from build123d import *

# Parameters (mm, degrees)
F0_R     = 5
F1_DEPTH = 10
F2_R     = 1.25
F3_DEPTH = 3.5
F4_R     = 10
F4_R_2   = 1.5
F4_R_3   = 5
F5_DEPTH = 3


with BuildPart() as f1:
    # F0 (on Top) → F1 (new body)
    with BuildSketch(Plane.XY):
        Circle(F0_R)
        with BuildLine():
            ThreePointArc((1.5, 2), (2.2360679775, 1.1180339887), (2.5, 0))
            ThreePointArc((2.5, 0), (2.2360679775, -1.1180339887), (1.5, -2))
            ThreePointArc((1.5, -2), (-2.5, 0), (1.5, 2))
        make_face(mode=Mode.SUBTRACT)
        with BuildLine():
            ThreePointArc((1.5, -2), (2.2360679775, -1.1180339887), (2.5, 0))
            ThreePointArc((2.5, 0), (2.2360679775, 1.1180339887), (1.5, 2))
            Line((1.5, 2), (1.5, -2))
        make_face()
    extrude(amount=F1_DEPTH)

    # F2 (on face) → F3 (cut, through all)
    with BuildSketch(Plane(origin=(1.5, 0, 0), x_dir=(0, -1, 0), z_dir=(-1, 0, 0))):
        with Locations((0, 5)):
            Circle(F2_R)
    extrude(amount=-F3_DEPTH, mode=Mode.SUBTRACT)

    # F4 (on face) → F5 (join)
    with BuildSketch(Plane.XY.offset(10)):
        Circle(F4_R)
        with Locations((0, -7.5)):
            Circle(F4_R_2, mode=Mode.SUBTRACT)
        with Locations((-7.5, 0)):
            Circle(F4_R_2, mode=Mode.SUBTRACT)
        Circle(F4_R_3, mode=Mode.SUBTRACT)
        with Locations((7.5, 0)):
            Circle(F4_R_2, mode=Mode.SUBTRACT)
        with Locations((0, 7.5)):
            Circle(F4_R_2, mode=Mode.SUBTRACT)
        Circle(F4_R_3)
        with BuildLine():
            Line((1.5, 2), (1.5, -2))
            ThreePointArc((1.5, -2), (-2.5, 0), (1.5, 2))
        make_face(mode=Mode.SUBTRACT)
        with BuildLine():
            ThreePointArc((1.5, 2), (-2.5, 0), (1.5, -2))
            Line((1.5, -2), (1.5, 2))
        make_face()
    extrude(amount=F5_DEPTH)


solid = f1.part
Verification items for the finished model (mm, model axes). A direction names the side the tool comes from. Give positions to 0.01 mm unless a question says otherwise; leave off trailing zeros. Order: outer loops, then holes, each group sorted by start corner. A loop starts at its lowest first (then second) coordinate and runs counter-clockwise, first axis right, second up. Notation, with made-up numbers: M 7.25,75.5 L 18.25,75.5 A17 cw 18.25,93.5 Z; hole C 87,72 d1. An arc over 180 degrees is marked long. Answer as a JSON object with one key per item and string values. Group by question number.
1) Mould release check, pull along X, two halves, no side actions. Record for faces 4 (the face through (-1.08, -4.88, 4.93)), 5 (the face through (-1, 0, 10)), 6 (the face through (2, 5, 10)): released by +X, released by -X, zero draft, split by the parting line, or undercut.
2) Cross-section at D-D (x = 8.5). Enter the section's corners in (y, z).
3) Cross-section at C-C (y = -8). Enter the section's corners in (x, z).
4) Access from +Z, -Z, +X, -X, +Y, -Y to the whole of each face (thin tool, end or side, straight path). Record for faces 1 (the face through (6, 0, 11)), 2 (the face through (3.23, 0.27, 3.78)), 3 (the face through (1.5, 1.4, 4.9)).
5) Depth check by flat-ended pin: pin 1 Ø2.5 at (x, y) = (0, 7.5) entering from +Z; pin 2 Ø3 at (x, y) = (-0.5, 0.5) entering from -Z; pin 3 Ø2 at (y, z) = (-2, 11) entering from -X; pin 4 Ø1.5 at (x, z) = (4.5, 2.5) entering from +Y. Enter the tip coordinate at first touch or a pass-through.
6) Scan lines: line 1 along Y through (x, z) = (0, 12.3); line 2 along X through (y, z) = (-0.75, 10.5); line 3 along X through (y, z) = (-0.5, 10.5). Record each from-to range of solid material in increasing order. Write a range as [from, to].
7) Cross-section at A-A (x = 0). Enter the section's corners in (y, z), then the cut area to 3 significant figures.
8) Cross-section at B-B (y = 0). Enter the section's corners in (x, z).
Result sheet:
{
 "1": {"face 4": "split by the parting line", "face 5": "undercut", "face 6": "zero draft"},
 "2": {"outline": "M -5.27,10 L -1.12,10 L -1.12,13 L -5.27,13 Z; M 1.12,10 L 5.27,10 L 5.27,13 L 1.12,13 Z"},
 "3": {"outline": "M -6,10 L -1.41,10 L -1.41,13 L -6,13 Z; M 1.41,10 L 6,10 L 6,13 L 1.41,13 Z"},
 "4": {"face 1": "+Z, -Z", "face 2": "+X", "face 3": "-Z"},
 "5": {"pin 1": "passes through", "pin 2": "stops at z = 10", "pin 3": "stops at x = -9.95", "pin 4": "stops at y = 3.31"},
 "6": {"line 1": "y = [-10, -9], [-6, 6], [9, 10]", "line 2": "x = [-9.97, -8.8], [-6.2, 6.2], [8.8, 9.97]", "line 3": "x = [-9.99, -8.91], [-6.09, 6.09], [8.91, 9.99]"},
 "7": {"outline": "M -10,10 L -9,10 L -9,13 L -10,13 Z; M -6,10 L -5,10 L -5,0 L -2.5,0 L -2.5,10 L 2.5,10 L 2.5,0 L 5,0 L 5,10 L 6,10 L 6,13 L -6,13 Z; M 9,10 L 10,10 L 10,13 L 9,13 Z", "area": "92.0 mm2"},
 "8": {"outline": "M -10,10 L -9,10 L -9,13 L -10,13 Z; M -6,10 L -5,10 L -5,0 L -2.5,0 L -2.5,10 L 1.5,10 L 1.5,6.25 L 5,6.25 L 5,10 L 6,10 L 6,13 L -6,13 Z; M 1.5,0 L 5,0 L 5,3.75 L 1.5,3.75 Z; M 9,10 L 10,10 L 10,13 L 9,13 Z"}
}
